```python
from build123d import *

# Parameters (mm, degrees)
SKETCH2_R                       = 6
SKETCH2_W                       = 16
SKETCH2_H                       = 9
BOSS_EXTRUDE1_DEPTH             = 22
BOSS_EXTRUDE2_START             = -10
SKETCH2_9_R                     = 6
BOSS_EXTRUDE2_DEPTH             = 10
CUT_EXTRUDE1_START              = -2
SKETCH3_R                       = 6
CUT_EXTRUDE1_DEPTH              = 2
SKETCH5_W                       = 16
SKETCH5_H                       = 9
BOSS_EXTRUDE3_DEPTH             = 10
M6X1_0_TAPPED_HOLE1_D           = 6
M6X1_0_TAPPED_HOLE1_DEPTH       = 16
M6X1_0_TAPPED_HOLE1_CSINK_D     = 6.05
M6X1_0_TAPPED_HOLE1_CSINK_ANGLE = 90
M6X1_0_TAPPED_HOLE1_TIP         = 1.732050808
HOLE1_D                         = 6
HOLE1_DEPTH                     = 15
HOLE1_CBORE_D                   = 10
HOLE1_CBORE_DEPTH               = 4


with BuildPart() as part:
    # Sketch2 → Boss-Extrude1 (new body)
    # profile 1 of 2: a face of its own
    with BuildSketch(Plane.XY):
        with BuildLine():
            Line((-32, 26), (-32, 16))
            Line((-32, 16), (-8, 16))
            Line((-8, 16), (8, 16))
            Line((8, 16), (32, 16))
            Line((32, 16), (32, 26))
            Line((32, 26), (27.5, 26))
            ThreePointArc((27.5, 26), (26.084330962, 26.355027189), (25.003729255, 27.336079218))
            Line((25.003729255, 27.336079218), (13.313443971, 44.874244172))
            ThreePointArc((13.313443971, 44.874244172), (7.550234872, 50.106521661), (0, 52))
            ThreePointArc((0, 52), (-7.550234872, 50.106521661), (-13.313443971, 44.874244172))
            Line((-13.313443971, 44.874244172), (-25.003729255, 27.336079218))
            ThreePointArc((-25.003729255, 27.336079218), (-26.084330962, 26.355027189), (-27.5, 26))
            Line((-27.5, 26), (-32, 26))
        make_face()
        with Locations((0, 36)):
            Circle(SKETCH2_R, mode=Mode.SUBTRACT)
    # profile 2 of 2: a face of its own
    with BuildSketch(Plane.XY):
        with Locations((0, 11.5)):
            Rectangle(SKETCH2_W, SKETCH2_H)
    extrude(amount=BOSS_EXTRUDE1_DEPTH)

    # Sketch2<9> → Boss-Extrude2 (add)
    # profile 1 of 4: a face of its own
    with BuildSketch(Plane.XY.offset(BOSS_EXTRUDE2_START)):
        with BuildLine():
            Line((32, 52), (0, 52))
            ThreePointArc((0, 52), (7.550234872, 50.106521661), (13.313443971, 44.874244172))
            Line((13.313443971, 44.874244172), (25.003729255, 27.336079218))
            ThreePointArc((25.003729255, 27.336079218), (26.084330962, 26.355027189), (27.5, 26))
            Line((27.5, 26), (32, 26))
            Line((32, 26), (32, 52))
        make_face()
    # profile 2 of 4: a face of its own
    with BuildSketch(Plane.XY.offset(BOSS_EXTRUDE2_START)):
        with BuildLine():
            Line((-32, 26), (-32, 16))
            Line((-32, 16), (-8, 16))
            Line((-8, 16), (8, 16))
            Line((8, 16), (32, 16))
            Line((32, 16), (32, 26))
            Line((32, 26), (27.5, 26))
            ThreePointArc((27.5, 26), (26.084330962, 26.355027189), (25.003729255, 27.336079218))
            Line((25.003729255, 27.336079218), (13.313443971, 44.874244172))
            ThreePointArc((13.313443971, 44.874244172), (7.550234872, 50.106521661), (0, 52))
            ThreePointArc((0, 52), (-7.550234872, 50.106521661), (-13.313443971, 44.874244172))
            Line((-13.313443971, 44.874244172), (-25.003729255, 27.336079218))
            ThreePointArc((-25.003729255, 27.336079218), (-26.084330962, 26.355027189), (-27.5, 26))
            Line((-27.5, 26), (-32, 26))
        make_face()
        with Locations((0, 36)):
            Circle(SKETCH2_9_R, mode=Mode.SUBTRACT)
    # profile 3 of 4: a face of its own
    with BuildSketch(Plane.XY.offset(BOSS_EXTRUDE2_START)):
        with BuildLine():
            Line((-32, 52), (-32, 26))
            Line((-32, 26), (-27.5, 26))
            ThreePointArc((-27.5, 26), (-26.084330962, 26.355027189), (-25.003729255, 27.336079218))
            Line((-25.003729255, 27.336079218), (-13.313443971, 44.874244172))
            ThreePointArc((-13.313443971, 44.874244172), (-7.550234872, 50.106521661), (0, 52))
            Line((0, 52), (-32, 52))
        make_face()
    # profile 4 of 4: a face of its own
    with BuildSketch(Plane.XY.offset(BOSS_EXTRUDE2_START)):
        with Locations((0, 36)):
            Circle(SKETCH2_9_R)
    extrude(amount=BOSS_EXTRUDE2_DEPTH)

    # Sketch3 → Cut-Extrude1 (cut)
    with BuildSketch(Plane.XY.offset(CUT_EXTRUDE1_START)):
        with Locations((0, 36)):
            Circle(SKETCH3_R)
    extrude(amount=CUT_EXTRUDE1_DEPTH, mode=Mode.SUBTRACT)

    # Sketch5 → Boss-Extrude3 (add)
    with BuildSketch(Plane(origin=(0, 0, 0), x_dir=(-1, 0, 0), z_dir=(0, 0, -1))):
        with Locations((0, 11.5)):
            Rectangle(SKETCH5_W, SKETCH5_H)
    extrude(amount=BOSS_EXTRUDE3_DEPTH)

    # M6x1.0 Tapped Hole1
    with Locations(Plane(origin=(0, 7, 14), x_dir=(-1, 0, 0), z_dir=(0, -1, 0))):
        with Locations((0, 0), (0, 16)):
            CounterSinkHole(M6X1_0_TAPPED_HOLE1_D / 2, M6X1_0_TAPPED_HOLE1_CSINK_D / 2, depth=M6X1_0_TAPPED_HOLE1_DEPTH, counter_sink_angle=M6X1_0_TAPPED_HOLE1_CSINK_ANGLE)
            with Locations((0, 0, -(M6X1_0_TAPPED_HOLE1_DEPTH + M6X1_0_TAPPED_HOLE1_TIP / 2))):  # 120° drill point
                Cone(0, M6X1_0_TAPPED_HOLE1_D / 2, M6X1_0_TAPPED_HOLE1_TIP, mode=Mode.SUBTRACT)

    # Hole1
    with Locations(Plane(origin=(0, 52, 10), x_dir=(1, 0, 0), z_dir=(0, 1, 0))):
        with Locations((0, 0)):
            CounterBoreHole(HOLE1_D / 2, HOLE1_CBORE_D / 2, HOLE1_CBORE_DEPTH, depth=HOLE1_DEPTH)


solid = part.part
```
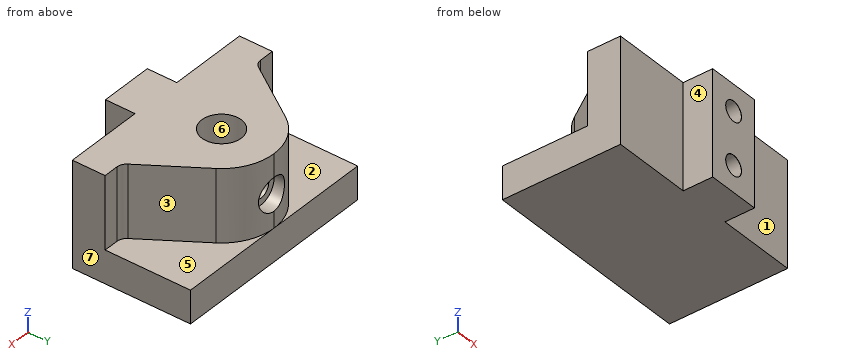
Check sheet for the modelled part. Datum: model origin and axes. Units: mm. Face numbers are marked on the shaded views. A direction names the side the tool comes from. Coordinates: 2 decimals unless noted, no trailing zeros. Loops run counter-clockwise (first coordinate to the right, second up) from the corner with the lowest first, then second, coordinate; pieces in that order, holes last.
1) Access from +Z, -Z, +X, -X, +Y, -Y to the whole of each face (thin tool, end or side, straight path). Record for the marked faces 1, 2, 3 and 4.
2) Sectioned sample at B-B (z = 2). Record the boundary of the cut face in (x, y).
3) Material ranges on probe 1 along Z at (x, y) = (0, 16.5); probe 2 along Z at (x, y) = (0, 43.5); probe 3 along X at (y, z) = (13, 14), recorded low to high.
4) Release check for a two-part mould opening along X. For the marked faces 5, 6 and 7 record: released by +X, released by -X, zero draft, split by the parting line, or undercut.
5) Gauge pin test, flat ends, axial feed: pin 1 (5 mm diameter, centred on x = 1, z = 12.5, fed in from +Y); pin 2 (12 mm diameter, centred on x = -16.5, z = 9, fed in from -Y); pin 3 (1.3 mm diameter, centred on x = 29.5, z = 11, fed in from +Y). Record the tip position at first contact, or that the pin passes through.
6) Sectioned sample at A-A (y = 13). Record the boundary of the cut face in (x, z), and give its area (3 significant figures).
7) Sectioned sample at D-D (y = 32). Record the boundary of the cut face in (x, z).
8) Sectioned sample at C-C (x = -14.5). Record the boundary of the cut face in (y, z), and give its area (3 significant figures).
Check sheet entries:
1. face 1: +Z, -Z, +X, -Y
1. face 2: +Z, -X, +Y
1. face 3: +Z, +X, +Y
1. face 4: +Z, -Z, -X, -Y
2. outline: (-32, 16) - (-8, 16) - (-8, 7) - (8, 7) - (8, 16) - (32, 16) - (32, 26) - (27.5, 26) arc R3 cw to (25, 27.34) - (13.31, 44.87) arc R16 ccw to (-13.31, 44.87) - (-25, 27.34) arc R3 cw to (-27.5, 26) - (-32, 26) - close; hole circle Ø12 at (0, 36)
3. probe 1: z = -10 to -5, 1 to 11, 17 to 22
3. probe 2: z = -10 to 7, 13 to 22
3. probe 3: x = -8 to -3, 3 to 8
4. face 5: zero draft
4. face 6: undercut
4. face 7: released by +X
5. pin 1: stops at y = 51.99
5. pin 2: stops at y = 16
5. pin 3: stops at y = 26
6. outline: (-8, -10) - (8, -10) - (8, 22) - (-8, 22) - close; hole circle Ø6 at (0, -2); hole circle Ø6 at (0, 14)
6. area: 455 mm2
7. outline: (-32, -10) - (32, -10) - (32, 0) - (21.89, 0) - (21.89, 22) - (4.47, 22) - (4.47, -2) - (-4.47, -2) - (-4.47, 22) - (-21.89, 22) - (-21.89, 0) - (-32, 0) - close
8. outline: (16, -10) - (52, -10) - (52, 0) - (43.09, 0) - (43.09, 22) - (16, 22) - close
8. area: 956 mm2
